from build123d import *

# Parameters (mm, degrees)
F1_DEPTH = 12.7


with BuildPart() as f1:
    # F0 (on Top) → F1 (new body)
    with BuildSketch(Plane.XY):
        with BuildLine():
            ThreePointArc((-4.691688, 22.048172), (0, 22.541824), (4.691688, 22.048172))
            Line((4.691688, 22.048172), (4.691688, 36.896243))
            ThreePointArc((4.691688, 36.896243), (3.338552, 40.348328), (0, 41.96138))
            ThreePointArc((0, 41.96138), (-3.338552, 40.348328), (-4.691688, 36.896243))
            Line((-4.691688, 36.896243), (-4.691688, 22.048172))
        make_face()
        with BuildLine():
            ThreePointArc((-4.691688, 22.048172), (-14.184051, -17.519889), (22.541824, 0))
            ThreePointArc((22.541824, 0), (17.519889, 14.184051), (4.691688, 22.048172))
            ThreePointArc((4.691688, 22.048172), (0, 22.541824), (-4.691688, 22.048172))
        make_face()
    extrude(amount=F1_DEPTH)


solid = f1.part
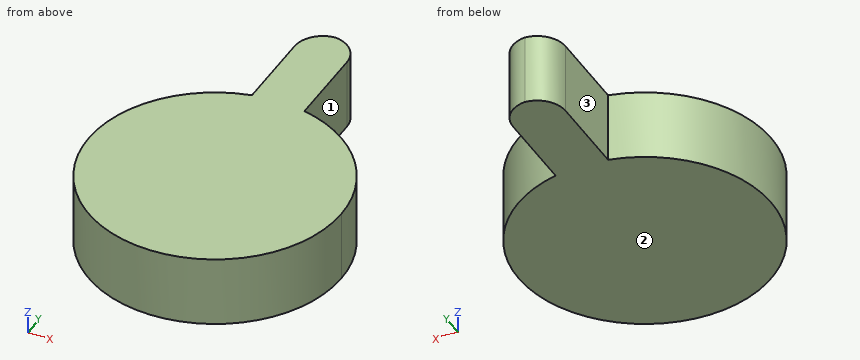
The model under review builds one solid part; all positions refer to its coordinate system, in mm. Face numbers are marked on the shaded views. A direction names the side the tool comes from. Round coordinates to 2 decimals unless told otherwise and drop trailing zeros. Write each loop counter-clockwise with the first axis right and the second up, starting at its lowest first coordinate (ties: lowest second). Pieces come first, ordered by that corner, then holes. Notation, with made-up numbers: (-19.75, 51) - (8.25, 51) arc R8 cw to (8.25, 61) - close; hole circle Ø6 at (78, -35). An arc over 180 degrees is marked (long way). One line per item, written item: value. Start each with the question number.
1. Consider section C-C on x = 16. Write out the cut boundary in (y, z), and give its area (3 significant figures).
2. Clearance check with flat-ended pins moving along their axes: P1, Ø4, axis at y = 30.5, z = 7.5, coming from the -X side; P2, Ø2, axis at x = 7.5, y = -9, coming from the -Z side; P3, Ø2, axis at y = -11.5, z = 1.5, coming from the +X side; P4, Ø5, axis at y = -15.5, z = 8, coming from the +X side. State where each tip first meets the part, or that it passes through.
3. Machinability: for the marked faces 1, 2 and 3, which of the approach directions +Z, -Z, +X, -X, +Y, -Y give a long, thin tool a straight path to every point of the face, cutting with its end or side? Answer none if there is none.
4. Consider section A-A on y = 27. Write out the cut boundary in (x, z), and give its area (3 significant figures).
5. To check wall thickness, follow L1, parallel to X at y = 30, z = 4.5; L2, parallel to Y at x = -18, z = 4.75; L3, parallel to X at y = 11, z = 3.75. State the ranges of each line that lie inside material, in increasing order. Write a range as from..to.
6. Consider section B-B on z = 7.75. Write out the cut boundary in (x, y).
Checks:
1. outline: (-15.88, 0) - (15.88, 0) - (15.88, 12.7) - (-15.88, 12.7) - close
1. area: 403 mm^2
2. P1: stops at x = -4.69
2. P2: stops at z = 0
2. P3: stops at x = 19.95
2. P4: stops at x = 18.42
3. face 1: +Z, -Z, +X, +Y
3. face 2: -Z, +X, -X, +Y, -Y
3. face 3: +Z, -Z, -X, +Y
4. outline: (-4.69, 0) - (4.69, 0) - (4.69, 12.7) - (-4.69, 12.7) - close
4. area: 119 mm^2
5. L1: x = -4.69..4.69
5. L2: y = -13.57..13.57
5. L3: x = -19.68..19.68
6. outline: (-4.69, 22.05) arc R22.54 ccw (long way) to (22.54, 0) arc R22.54 ccw to (4.69, 22.05) - (4.69, 36.9) arc R5.08 ccw to (0, 41.96) arc R5.08 ccw to (-4.69, 36.9) - close
